Job drawing, mm, ordinate dimensions from the low corner. One solid piece. Give positions to 0.01 mm unless a question says otherwise; leave off trailing zeros. Order: outer loops, then holes, each group sorted by start corner. A loop starts at its lowest first (then second) coordinate and runs counter-clockwise, first axis right, second up.
1. Slice it at D-D on x = 42.5. List the corners of the cut face in (y, z).
2. Slice it at B-B on x = 25. List the corners of the cut face in (y, z), and give its area (3 significant figures).
3. Slice it at C-C on z = 22. List the corners of the cut face in (x, y).
4. Drop flat-ended pins along their axis: pin 1 Ø12 at (y, z) = (24, 5.5) entering from -X; pin 2 Ø4 at (x, y) = (41, 15) entering from -Z; pin 3 Ø1.2 at (x, z) = (7.5, 29.5) entering from +Y. Give the stop position or say it passes through.
5. Mould opens along Y. For the marked faces 1, 2, 3 and 4 say: +Y half, -Y half, draft (parallel to the pull), parting line (faces both ways), or undercut.
6. Slice it at A-A on y = 15. List the corners of the cut face in (x, z), and give its area (3 significant figures).
7. Probe line 1 (Z direction, x = 8.5, y = 21.5); line 2 (X direction, y = 25.5, z = 6) (1 decimal); line 3 (X direction, y = 15.5, z = 31.5). List the from-to ranges inside material, lowest first.
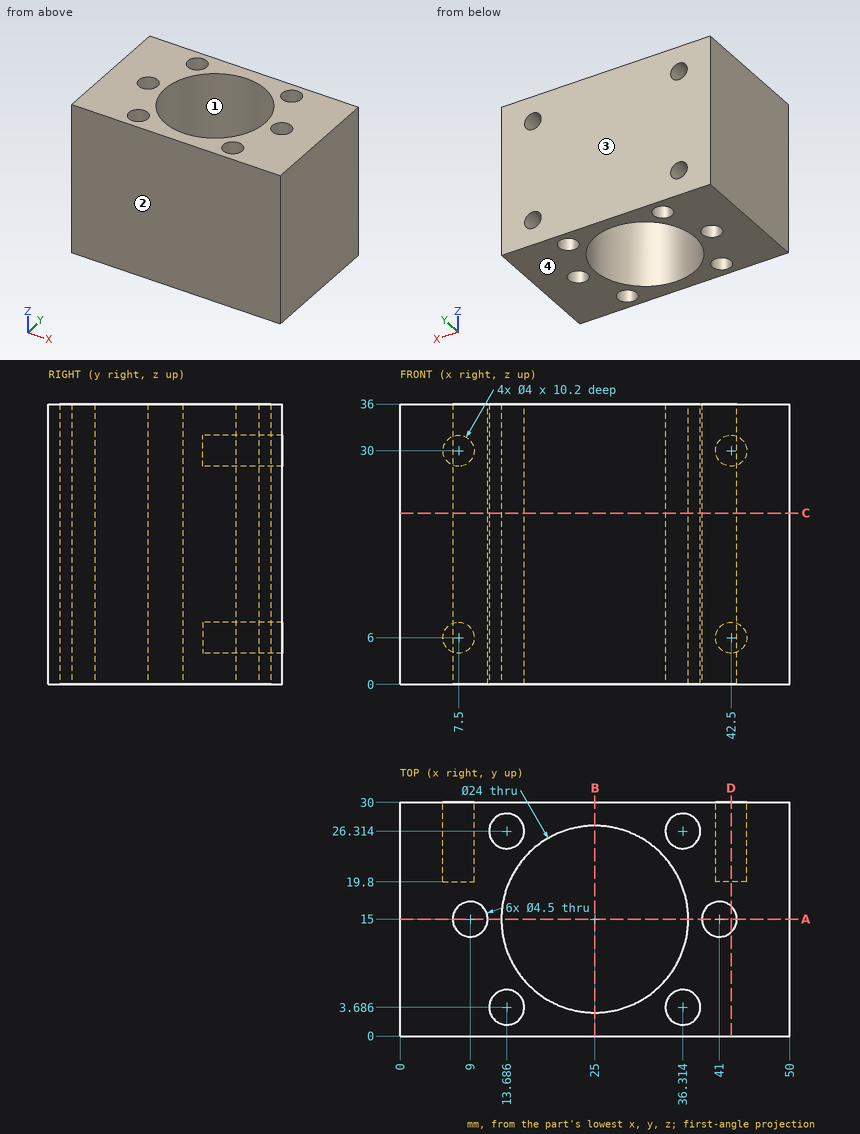
Data:
1. outline: (0, 0) - (13.32, 0) - (13.32, 36) - (0, 36) - close; (16.68, 0) - (30, 0) - (30, 4) - (19.8, 4) - (19.8, 8) - (30, 8) - (30, 28) - (19.8, 28) - (19.8, 32) - (30, 32) - (30, 36) - (16.68, 36) - close
2. outline: (0, 0) - (3, 0) - (3, 36) - (0, 36) - close; (27, 0) - (30, 0) - (30, 36) - (27, 36) - close
2. area: 216 mm2
3. outline: (0, 0) - (50, 0) - (50, 30) - (0, 30) - close; hole circle Ø4.5 at (9, 15); hole circle Ø4.5 at (13.69, 3.69); hole circle Ø4.5 at (13.69, 26.31); hole circle Ø24 at (25, 15); hole circle Ø4.5 at (36.31, 3.69); hole circle Ø4.5 at (36.31, 26.31); hole circle Ø4.5 at (41, 15)
4. pin 1: stops at x = 0
4. pin 2: passes through
4. pin 3: stops at y = 19.8
5. face 1: undercut
5. face 2: -Y half
5. face 3: +Y half
5. face 4: draft
6. outline: (0, 0) - (6.75, 0) - (6.75, 36) - (0, 36) - close; (11.25, 0) - (13, 0) - (13, 36) - (11.25, 36) - close; (37, 0) - (38.75, 0) - (38.75, 36) - (37, 36) - close; (43.25, 0) - (50, 0) - (50, 36) - (43.25, 36) - close
6. area: 612 mm2
7. line 1: z = 0 to 4.27, 7.73 to 28.27, 31.73 to 36
7. line 2: x = 0 to 5.5, 9.5 to 11.6, 15.8 to 19.2, 30.8 to 34.2, 38.4 to 40.5, 44.5 to 50
7. line 3: x = 0 to 6.81, 11.19 to 13.01, 36.99 to 38.81, 43.19 to 50
